Answer from the drawing. Dimensions are ordinates in mm from the lowest x, y and z of the part. Give positions to 0.01 mm unless a question says otherwise; leave off trailing zeros. Loops run counter-clockwise (first coordinate to the right, second up) from the corner with the lowest first, then second, coordinate; pieces in that order, holes last. Notation, with made-up numbers: (-7.75, 20.5) -> (32.25, 20.5) arc R19 cw to (32.25, 43.5) -> close; hole circle Ø9 at (79, 17.25). An arc over 180 degrees is marked (long way). Return JSON: item names as keys, results as strings. Group by question number.
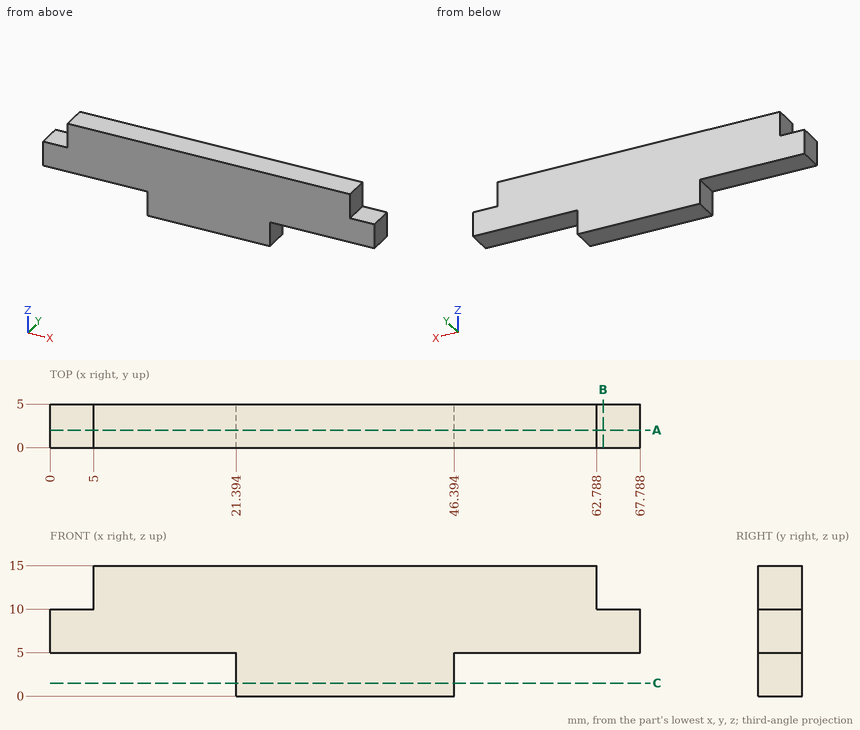
1. Section C-C on z = 1.5 is taken. Determine the outline of the cut face in (x, y).
2. Flat-ended cylindrical pins translate along their axes: pin 1 Ø2.5 at (x, y) = (60.5, 3) entering from -Z; pin 2 Ø1 at (y, z) = (2, 11) entering from +X; pin 3 Ø2.5 at (y, z) = (1.5, 12.5) entering from -X. Find the tip coordinate at first contact, or state that the pin passes through.
3. Section A-A on y = 2 is taken. Determine the outline of the cut face in (x, z).
4. Section B-B on x = 63.5 is taken. Determine the outline of the cut face in (y, z), then the cut area to 3 significant figures.
5. Straight lines are drawn through the part: line 1 (Z direction, x = 54.5, y = 3.25); line 2 (X direction, y = 2.7, z = 12); line 3 (X direction, y = 1.4, z = 4.5). For each, find the intervals that lie inside material, in ascending order. Write a range as from..to.
Completed:
{
 "1": {"outline": "(21.39, 0) -> (46.39, 0) -> (46.39, 5) -> (21.39, 5) -> close"},
 "2": {"pin 1": "stops at z = 5", "pin 2": "stops at x = 62.79", "pin 3": "stops at x = 5"},
 "3": {"outline": "(0, 5) -> (21.39, 5) -> (21.39, 0) -> (46.39, 0) -> (46.39, 5) -> (67.79, 5) -> (67.79, 10) -> (62.79, 10) -> (62.79, 15) -> (5, 15) -> (5, 10) -> (0, 10) -> close"},
 "4": {"outline": "(0, 5) -> (5, 5) -> (5, 10) -> (0, 10) -> close", "area": "25.0 mm²"},
 "5": {"line 1": "z = 5..15", "line 2": "x = 5..62.79", "line 3": "x = 21.39..46.39"}
}
